Print and shaded views of the part. All mm, measured from the part's lowest x, y and z. A direction names the side the tool comes from. Round coordinates to 2 decimals unless told otherwise and drop trailing zeros. Loops run counter-clockwise (first coordinate to the right, second up) from the corner with the lowest first, then second, coordinate; pieces in that order, holes last. Notation, with made-up numbers: (78.25, 63.5) - (95.25, 63.5) arc R14 cw to (95.25, 76.5) - close; hole circle Ø3 at (-9.75, 52). An arc over 180 degrees is marked (long way). Use one line per item in the form item = value.
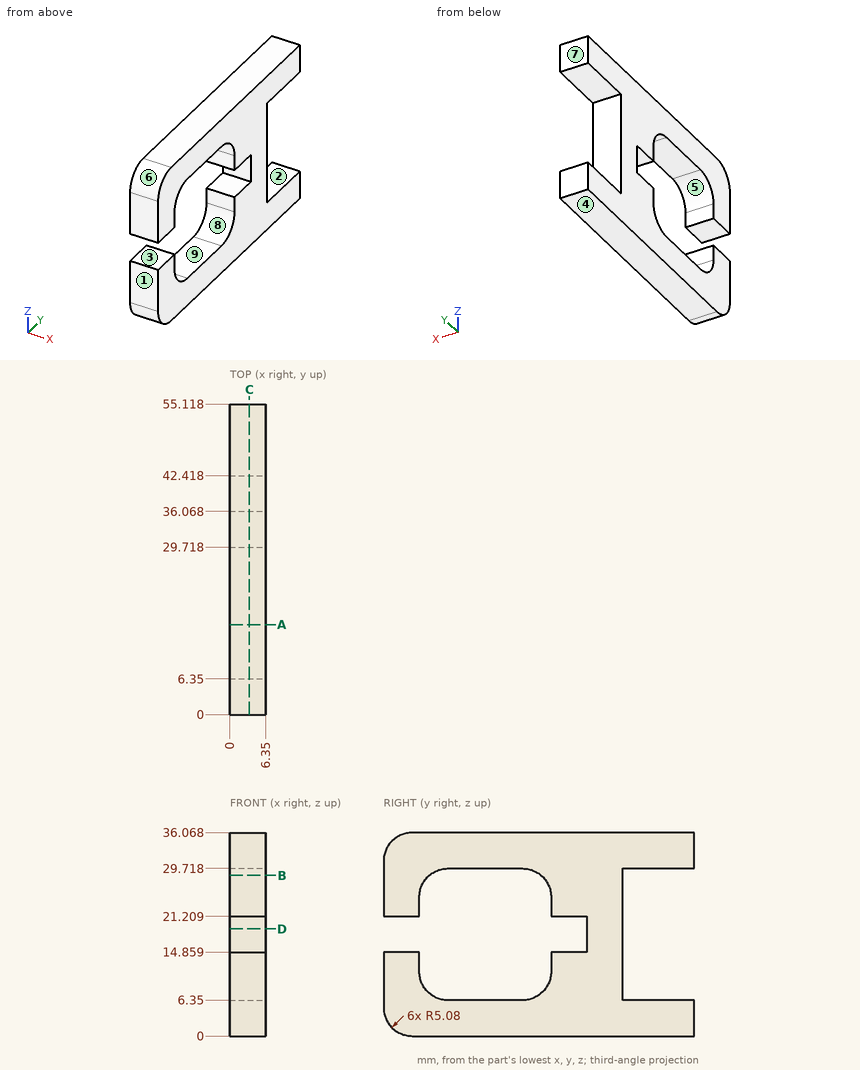
1. Cut at B-B, the plane z = 28.5. Give the cut face in (x, y).
Geometry check:
outline = (0, 0) - (6.35, 0) - (6.35, 8.13) - (0, 8.13) - close; (0, 27.94) - (6.35, 27.94) - (6.35, 42.42) - (0, 42.42) - close
2. Cut at C-C, the plane x = 3.5. Give the cut face in (y, z), plus the area to 3 significant figures.
Geometry check:
outline = (0, 5.08) arc R5.08 ccw to (5.08, 0) - (55.12, 0) - (55.12, 6.35) - (42.42, 6.35) - (42.42, 29.72) - (55.12, 29.72) - (55.12, 36.07) - (5.08, 36.07) arc R5.08 ccw to (0, 30.99) - (0, 21.21) - (6.35, 21.21) - (6.35, 24.64) arc R5.08 cw to (11.43, 29.72) - (24.64, 29.72) arc R5.08 cw to (29.72, 24.64) - (29.72, 21.21) - (36.07, 21.21) - (36.07, 14.86) - (29.72, 14.86) - (29.72, 11.43) arc R5.08 cw to (24.64, 6.35) - (11.43, 6.35) arc R5.08 cw to (6.35, 11.43) - (6.35, 14.86) - (0, 14.86) - close
area = 1,080 mm^2
3. Cut at D-D, the plane z = 19. Give the cut face in (x, y).
Geometry check:
outline = (0, 36.07) - (6.35, 36.07) - (6.35, 42.42) - (0, 42.42) - close
4. Wall check: probe 1 along Z at (x, y) = (2, 15); probe 2 along Z at (x, y) = (3.5, 31.5); probe 3 along Y at (x, z) = (3, 17). Give the ranges that are in metal, low to high.
Geometry check:
probe_1 = 0 to 6.35, 29.72 to 36.07
probe_2 = 0 to 14.86, 21.21 to 36.07
probe_3 = 36.07 to 42.42
5. Tool access for the marked faces 1, 2, 3, 4 and 5: list every direction of +Z, -Z, +X, -X, +Y, -Y with a clear straight run to the whole face (end or side of a thin tool).
Geometry check:
face_1 = +Z, -Z, +X, -X, -Y
face_2 = +X, -X, +Y
face_3 = +X, -X, -Y
face_4 = -Z, +X, -X, +Y, -Y
face_5 = +X, -X
6. Cut at A-A, the plane y = 16. Give the cut face in (x, z), plus the area to 3 significant figures.
Geometry check:
outline = (0, 0) - (6.35, 0) - (6.35, 6.35) - (0, 6.35) - close; (0, 29.72) - (6.35, 29.72) - (6.35, 36.07) - (0, 36.07) - close
area = 80.6 mm^2
7. Pull direction Y, two halves, no side cores. Call the marked faces 6, 7, 8 and 9: +Y half, -Y half, draft (parallel to the pull), parting line (faces both ways), or undercut.
Geometry check:
face_6 = -Y half
face_7 = +Y half
face_8 = undercut
face_9 = undercut
8. Flat gauge pins, fed straight in: pin 1 (1.9 mm diameter, centred on x = 2.5, y = 1.5, fed in from -Z); pin 2 (2.5 mm diameter, centred on x = 2.5, z = 14, fed in from +Y); pin 3 (3 mm diameter, centred on x = 4, z = 17.5, fed in from -Y); pin 4 (3 mm diameter, centred on y = 8.5, z = 27, fed in from -X). Where does each tip first touch, or does it go through?
Geometry check:
pin_1 = 0.73
pin_2 = 42.42
pin_3 = 36.07
pin_4 = 0
